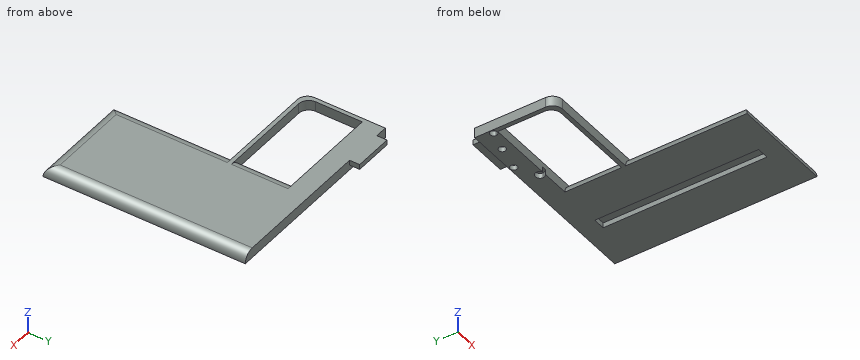
from build123d import *

# Parameters (mm, degrees)
F0_W     = 48
F0_H     = 10
F1_DEPTH = 5
F2_R     = 4.99999
F3_R     = 5
F4_W     = 6
F4_H     = 81
F4_R     = 1.75
F5_DEPTH = 2.5
F6_W     = 19.5
F6_H     = 2.5
F7_DEPTH = 5


# Not quite as in the source:
# - a fillet or chamfer is up to 0.001 mm smaller than in the source, because OpenCascade refuses the exact size


with BuildPart() as f1:
    # F0 (on Top) → F1 (new body)
    with BuildSketch(Plane.XY):
        Polygon((-73, 40), (-73, 50), (-75, 50), (-75, 10), (-25, 10), (-25, 12), (-73, 12), align=None)
        Polygon((25, -50), (25, 50), (-25, 50), (-25, 40), (-25, 12), (-25, 10), (-25, -50), align=None)
        with Locations((-49, 45)):
            Rectangle(F0_W, F0_H)
    extrude(amount=-F1_DEPTH)

    # F2 (radius 5 in the source; OpenCascade refuses exactly that, so slightly less here)
    f2_edges = [f1.edges().sort_by_distance(p)[0] for p in [
        (-25, -20, 0),
        (0, -50, 0),
        (25, 0, 0),
        (-25, 26, 0),
    ]]
    fillet(f2_edges, radius=F2_R)

    # F3
    f3_edges = [f1.edges().sort_by_distance(p)[0] for p in [
        (-73, 12, -2.5),
        (-75, 10, -2.5),
    ]]
    fillet(f3_edges, radius=F3_R)

    # F4 (on face) → F5 (cut)
    with BuildSketch(Plane(origin=(0, 0, -5), x_dir=(1, 0, 0), z_dir=(0, 0, -1))):
        Rectangle(F4_W, F4_H)
        with BuildLine():
            ThreePointArc((-41.0307764064, -40), (-41.1711646096, -43.9211646096), (-37.75, -42))
            ThreePointArc((-37.75, -42), (-38.0788353904, -40.8288353904), (-38.9692235936, -40))
            Line((-38.9692235936, -40), (-41.0307764064, -40))
        make_face()
        with Locations((-50, -48)):
            Circle(F4_R)
        with Locations((-62.5, -45)):
            Circle(F4_R)
        with BuildLine():
            ThreePointArc((-71.25, -42), (-71.7625631329, -40.7625631329), (-73, -40.25))
            ThreePointArc((-73, -40.25), (-74.2374368671, -43.2374368671), (-71.25, -42))
        make_face()
    extrude(amount=-F5_DEPTH, mode=Mode.SUBTRACT)

    # F6 (on face) → F7 (join)
    with BuildSketch(Plane(origin=(0, 50, 0), x_dir=(-1, 0, 0), z_dir=(0, 1, 0))):
        with Locations((59.25, -1.25)):
            Rectangle(F6_W, F6_H)
    extrude(amount=F7_DEPTH)


solid = f1.part
Could you check a few things on this model? Use its own coordinates, in mm. Give positions to 0.01 mm unless a question says otherwise; leave off trailing zeros. Order: outer loops, then holes, each group sorted by start corner. A loop starts at its lowest first (then second) coordinate and runs counter-clockwise, first axis right, second up. Notation, with made-up numbers: (50.25, 41) - (66.25, 41) arc R14 cw to (66.25, 62) - close; hole circle Ø10 at (-28.75, 89.25). An arc over 180 degrees is marked (long way). Return JSON: item names as keys, results as strings. Group by question number.
Q1. Will these pins go through, and if not, where does the flat tip stop? pin 1 Ø3 at (y, z) = (13, -0.5) entering from +X; pin 2 Ø1.2 at (x, z) = (0.5, -3) entering from -Y; pin 3 Ø7 at (x, y) = (-40, 42) entering from -Z; pin 4 Ø1.2 at (x, z) = (1, -4) entering from +Y.
Q2. Please list where these lines run through material, in increasing order: line 1 along Y through (x, z) = (-62.5, -4.45); line 2 along Y through (x, z) = (-50, -3.45); line 3 along X through (y, z) = (42, -4.1). Write a range as [from, to].
Q3. Suppose I cut it at A-A, the plane x = -62.5. Please give me the cut outline in (y, z), and give its area (4 significant figures).
Resolved:
{
 "1": {"pin 1": "stops at x = 24", "pin 2": "stops at y = -49.8", "pin 3": "stops at z = -5", "pin 4": "stops at y = 50"},
 "2": {"line 1": "y = [10, 12], [40, 43.25], [46.75, 50]", "line 2": "y = [10, 12], [40, 46.25], [49.75, 50]", "line 3": "x = [-75, -74.75], [-71.25, -42.25], [-37.75, 24.92]"},
 "3": {"outline": "(10, -5) - (12, -5) - (12, 0) - (10, 0) - close; (40, -5) - (43.25, -5) - (43.25, -2.5) - (46.75, -2.5) - (46.75, -5) - (50, -5) - (50, -2.5) - (55, -2.5) - (55, 0) - (40, 0) - close", "area": "63.75 mm2"}
}
